Input: dimensioned drawing with shaded views. Units: mm. Origin: part minimum x, y, z. Give positions to 0.01 mm unless a question says otherwise; leave off trailing zeros. Write each loop counter-clockwise with the first axis right and the second up, starting at its lowest first coordinate (ties: lowest second). Pieces come first, ordered by that corner, then holes. Notation, with made-up numbers: (70, 57) -> (104, 57) arc R29 cw to (104, 89) -> close; hole circle Ø7 at (13, 13.25). An arc over 180 degrees is marked (long way). Answer as a JSON object with one key per item and string values.
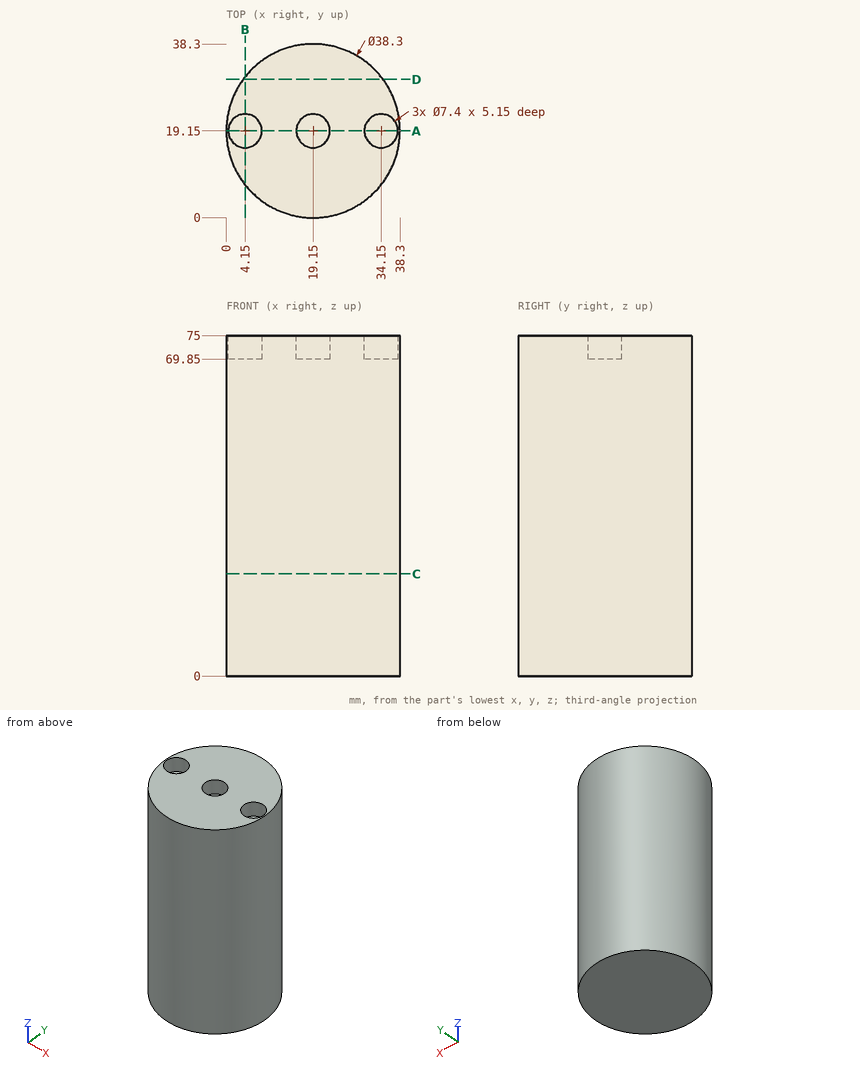
Q1. Cut plane B-B (x = 4.15). Return the cut outline in (y, z), and give its area (3 significant figures).
Values:
{"outline": "(7.25, 0) -> (31.05, 0) -> (31.05, 75) -> (22.85, 75) -> (22.85, 69.85) -> (15.45, 69.85) -> (15.45, 75) -> (7.25, 75) -> close", "area": "1,750 mm²"}
Q2. First-contact query: P1, Ø6, axis at y = 26, z = 35.5, coming from the +X side; P2, Ø6, axis at x = 19.15, y = 19.15, coming from the +Z side; P3, Ø2, axis at x = 15, z = 18, coming from the +Y side. Flat tips, straight axial feed; report the tip coordinate or a pass-through.
Values:
{"P1": "x = 37.91", "P2": "z = 69.85", "P3": "y = 38.04"}
Q3. Cut plane A-A (y = 19.15). Return the cut outline in (x, z), and give its area (3 significant figures).
Values:
{"outline": "(0, 0) -> (38.3, 0) -> (38.3, 75) -> (37.85, 75) -> (37.85, 69.85) -> (30.45, 69.85) -> (30.45, 75) -> (22.85, 75) -> (22.85, 69.85) -> (15.45, 69.85) -> (15.45, 75) -> (7.85, 75) -> (7.85, 69.85) -> (0.45, 69.85) -> (0.45, 75) -> (0, 75) -> close", "area": "2,760 mm²"}
Q4. Cut plane D-D (y = 30.5). Return the cut outline in (x, z), and give its area (3 significant figures).
Values:
{"outline": "(3.73, 0) -> (34.57, 0) -> (34.57, 75) -> (3.73, 75) -> close", "area": "2,310 mm²"}
Q5. Material intervals for L1, parallel to X at y = 17, z = 71; L2, parallel to Y at x = 19.15, z = 73.75; L3, parallel to Y at x = 34, z = 73, sorted ascending. Write a range as from..to.
Values:
{"L1": "0.12..1.14, 7.16..16.14, 22.16..31.14, 37.16..38.18", "L2": "0..15.45, 22.85..38.3", "L3": "7.06..15.45, 22.85..31.24"}
Q6. Cut plane C-C (z = 22.5). Return the cut outline in (x, y), and give its area (3 significant figures).
Values:
{"outline": "circle Ø38.3 at (19.15, 19.15)", "area": "1,150 mm²"}
